CAD build for the part. Positions are in the model's coordinates, mm. Face numbers are marked on the shaded views. A direction names the side the tool comes from. Coordinates: 2 decimals unless noted, no trailing zeros. Loops run counter-clockwise (first coordinate to the right, second up) from the corner with the lowest first, then second, coordinate; pieces in that order, holes last. Notation, with made-up numbers: (-26, -9.75) -> (-4, -9.75) arc R29 cw to (-4, 21.25) -> close; hole circle Ø4 at (80, 58.25). An arc over 180 degrees is marked (long way). Write each question's results on one line, items separated by ' | '.
```python
from build123d import *

# Parameters (mm, degrees)
SKETCH1_R           = 4.25
BOSS_EXTRUDE1_DEPTH = 23
SKETCH2_R           = 5.25
BOSS_EXTRUDE2_DEPTH = 5
SKETCH6_R           = 1.5
CUT_EXTRUDE3_DEPTH  = 2
SKETCH7_R           = 1.75
CUT_EXTRUDE4_DEPTH  = 29.0000001
CUT_EXTRUDE5_DEPTH  = 4


with BuildPart() as part:
    # Sketch1 → Boss-Extrude1 (new body)
    with BuildSketch(Plane.XY):
        Circle(SKETCH1_R)
    extrude(amount=BOSS_EXTRUDE1_DEPTH)

    # Sketch2 → Boss-Extrude2 (add)
    with BuildSketch(Plane.XY.offset(23)):
        Circle(SKETCH2_R)
    extrude(amount=BOSS_EXTRUDE2_DEPTH)

    # Sketch6 → Cut-Extrude3 (cut)
    with BuildSketch(Plane(origin=(4.25, 0, 0), x_dir=(0, 0, -1), z_dir=(1, 0, 0))):
        with Locations((-3.5, 0)):
            Circle(SKETCH6_R)
    extrude(amount=-CUT_EXTRUDE3_DEPTH, mode=Mode.SUBTRACT)

    # Sketch7 → Cut-Extrude4 (cut, through all)
    with BuildSketch(Plane.XY.offset(28)):
        Circle(SKETCH7_R)
    extrude(amount=-CUT_EXTRUDE4_DEPTH, mode=Mode.SUBTRACT)

    # Sketch8 → Cut-Extrude5 (cut)
    with BuildSketch(Plane(origin=(0, 0, 0), x_dir=(-1, 0, 0), z_dir=(0, 0, -1))):
        Polygon((-0.22790745, 3.456596331), (-3.107453958, 1.530924524), (-2.879546508, -1.925671807), (0.22790745, -3.456596331), (3.107453958, -1.530924524), (2.879546508, 1.925671807), align=None)
    extrude(amount=-CUT_EXTRUDE5_DEPTH, mode=Mode.SUBTRACT)


solid = part.part
```
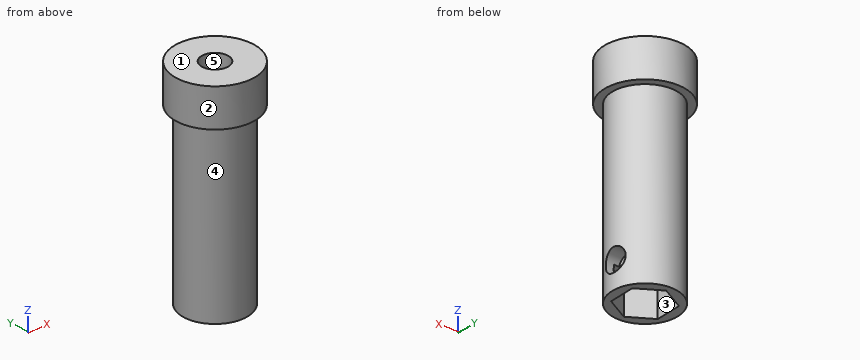
Q1. Cut at A-A on z = 1.5. Write the cut outline in (x, y).
Results are:
outline: circle Ø8.5 at (0, 0); hole (-3.11, -1.53) -> (-0.23, -3.46) -> (2.88, -1.93) -> (3.11, 1.53) -> (0.23, 3.46) -> (-2.88, 1.93) -> close
Q2. Cut at C-C on x = -2.5. Write the cut outline in (y, z), and give its area (3 significant figures).
Results are:
outline: (-4.62, 23) -> (-3.44, 23) -> (-3.44, 0) -> (-1.94, 0) -> (-1.94, 4) -> (2.11, 4) -> (2.11, 0) -> (3.44, 0) -> (3.44, 23) -> (4.62, 23) -> (4.62, 28) -> (-4.62, 28) -> close | area: 188 mm^2
Q3. Wall check: L1, parallel to Z at x = 3.85, y = 0; L2, parallel to Y at x = 0, z = 24.5; L3, parallel to Y at x = 0, z = 10.25. Give the ranges that are in metal, low to high. Write a range as from..to.
Results are:
L1: 0..2, 5..28 | L2: -5.25..-1.75, 1.75..5.25 | L3: -4.25..-1.75, 1.75..4.25
Q4. Cut at D-D on y = 3. Write the cut outline in (x, z), and give its area (3 significant figures).
Results are:
outline: (-4.31, 23) -> (-3.01, 23) -> (-3.01, 0) -> (-0.7, 0) -> (-0.7, 4) -> (0.91, 4) -> (0.91, 0) -> (3.01, 0) -> (3.01, 23) -> (4.31, 23) -> (4.31, 28) -> (-4.31, 28) -> close | area: 175 mm^2
Q5. Cut at B-B on y = 0. Write the cut outline in (x, z), and give its area (3 significant figures).
Results are:
outline: (-5.25, 23) -> (-4.25, 23) -> (-4.25, 0) -> (-3.01, 0) -> (-3.01, 4) -> (-1.75, 4) -> (-1.75, 28) -> (-5.25, 28) -> close; (1.75, 4) -> (2.25, 4) -> (2.25, 5) -> (4.25, 5) -> (4.25, 23) -> (5.25, 23) -> (5.25, 28) -> (1.75, 28) -> close; (3.01, 0) -> (4.25, 0) -> (4.25, 2) -> (3.01, 2) -> close | area: 135 mm^2
Q6. Which spindle directions (+Z, -Z, +X, -X, +Y, -Y) get a long thin tool onto all of the face, cutting with end or side? Do the marked faces 4 and 5. Say none if no direction does.
Results are:
face 4: -Z | face 5: +Z, -Z
Q7. Pull direction Y, two halves, no side cores. Call the marked faces 1, 2 and 3: +Y half, -Y half, draft (parallel to the pull), parting line (faces both ways), or undercut.
Results are:
face 1: draft | face 2: parting line | face 3: undercut
Q8. Drop flat-ended pins along their axis: pin 1 (3 mm diameter, centred on x = -2, z = 14.5, fed in from -Y); pin 2 (1.5 mm diameter, centred on y = 2, z = 24.5, fed in from -X); pin 3 (1 mm diameter, centred on y = -1, z = 21.5, fed in from +X). Give the stop position or say it passes through.
Results are:
pin 1: y = -4.22 | pin 2: x = -5.1 | pin 3: x = 4.22
